Build history of the part. All positions in model axes, mm. A direction names the side the tool comes from. Round coordinates to 2 decimals unless told otherwise and drop trailing zeros. Write each loop counter-clockwise with the first axis right and the second up, starting at its lowest first coordinate (ties: lowest second). Pieces come first, ordered by that corner, then holes.
from build123d import *

# Parameters (mm, degrees)
F1_DEPTH = 225
F2_T     = -2
F3_W     = 2
F3_H     = 58
F4_DEPTH = 446
F5_R     = 26.5
F6_DEPTH = 25.4
F7_R     = 27.5
F7_R_2   = 26.5
F8_DEPTH = 20


with BuildPart() as f1:
    # F0 (on Front) → F1 (new body, symmetric)
    with BuildSketch(Plane.XZ):
        with BuildLine():
            Line((0, 30), (0, 0))
            Line((0, 0), (140, 0))
            Line((140, 0), (140, 80))
            Line((140, 80), (50, 80))
            ThreePointArc((50, 80), (14.6446609407, 65.3553390593), (0, 30))
        make_face()
    extrude(amount=F1_DEPTH, both=True)

    # F2
    f2_openings = [f1.faces().sort_by_distance(p)[0] for p in [
        (140, 0, 40),
    ]]
    offset(amount=F2_T, openings=f2_openings)

    # F3 (on face) → F4 (join, through all)
    with BuildSketch(Plane.XZ.offset(-223)):
        with Locations((139, 31)):
            Rectangle(F3_W, F3_H)
    extrude(amount=F4_DEPTH)

    # F5 (on face) → F6 (cut)
    with BuildSketch(Plane(origin=(0, 0, 0), x_dir=(1, 0, 0), z_dir=(0, 0, -1))):
        with Locations((57, 175)):
            Circle(F5_R)
        with Locations((56.9928, -175)):
            Circle(F5_R)
    extrude(amount=-F6_DEPTH, mode=Mode.SUBTRACT)

    # F7 (on face) → F8 (join)
    with BuildSketch(Plane(origin=(0, 0, 0), x_dir=(1, 0, 0), z_dir=(0, 0, -1))):
        with Locations((57, 175)):
            Circle(F7_R)
        with Locations((57, 175)):
            Circle(F7_R_2, mode=Mode.SUBTRACT)
        with Locations((56.9928, -175)):
            Circle(F7_R)
        with Locations((56.9928, -175)):
            Circle(F7_R_2, mode=Mode.SUBTRACT)
    extrude(amount=F8_DEPTH)


solid = f1.part
1) Pin check, flat tips, straight feed: pin 1 Ø12 at (y, z) = (-174, -2) entering from -X; pin 2 Ø5 at (x, y) = (57.5, -144) entering from -Z. Stop position of each tip, or through.
Results:
pin 1: stops at x = 0
pin 2: stops at z = 0
2) Slice it at C-C (x = 125.5). Write the cut outline in (y, z).
Results:
outline: (-225, 0) - (225, 0) - (225, 80) - (-225, 80) - close; hole (-223, 2) - (223, 2) - (223, 78) - (-223, 78) - close
3) Wall check: L1, parallel to Z at x = 107, y = -3; L2, parallel to Y at x = 120.5, z = 42; L3, parallel to X at y = 113.5, z = 17.5. Give the ranges that are in metal, low to high.
Results:
L1: z = 0 to 2, 78 to 80
L2: y = -225 to -223, 223 to 225
L3: x = 0 to 2, 138 to 140
4) Slice it at A-A (y = 175). Write the cut outline in (x, z).
Results:
outline: (0, 0) - (29.49, 0) - (29.49, -20) - (30.49, -20) - (30.49, 2) - (2, 2) - (2, 30) arc R48 cw to (50, 78) - (140, 78) - (140, 80) - (50, 80) arc R50 ccw to (0, 30) - close; (83.49, -20) - (84.49, -20) - (84.49, 0) - (140, 0) - (140, 60) - (138, 60) - (138, 2) - (83.49, 2) - close
5) Which spindle directions (+Z, -Z, +X, -X, +Y, -Y) get a long thin tool onto all of the face, cutting with end or side? Do faces 4 (the cylindrical face through (29.52, 173.79, -9.86)), 5 (the flat face through (69, -3, 2)), 6 (the flat face through (0, -3, 15)). Say none if no direction does.
Results:
face 4: -Z
face 5: none
face 6: +Z, -Z, -X, +Y, -Y
6) Mould opens along X. For faces 1 (the cylindrical face through (35.177, -158.267, -9.86)), 2 (the flat face through (70, -223, 41)), 3 (the flat face through (96, -3, 78)) say: released by +X, released by -X, zero draft, split by the parting line, or undercut.
Results:
face 1: split by the parting line
face 2: undercut
face 3: zero draft
7) Slice it at D-D (z = 34). Write the cut outline in (x, y).
Results:
outline: (0.16, -225) - (140, -225) - (140, 225) - (0.16, 225) - close; hole (2.17, -223) - (138, -223) - (138, 223) - (2.17, 223) - close
8) Slice it at B-B (x = 57). Write the cut outline in (y, z).
Results:
outline: (-225, 0) - (-202.5, 0) - (-202.5, -20) - (-201.5, -20) - (-201.5, 2) - (-223, 2) - (-223, 78) - (223, 78) - (223, 2) - (201.5, 2) - (201.5, -20) - (202.5, -20) - (202.5, 0) - (225, 0) - (225, 80) - (-225, 80) - close; (-148.5, -20) - (-147.5, -20) - (-147.5, 0) - (147.5, 0) - (147.5, -20) - (148.5, -20) - (148.5, 2) - (-148.5, 2) - close
